Build history of the part. All positions in model axes, mm. A direction names the side the tool comes from. Give positions to 0.01 mm unless a question says otherwise; leave off trailing zeros. Write each loop counter-clockwise with the first axis right and the second up, starting at its lowest first coordinate (ties: lowest second). Pieces come first, ordered by that corner, then holes. Notation, with made-up numbers: (-13.75, 73) -> (28.25, 73) arc R16 cw to (28.25, 85) -> close; hole circle Ø1 at (-30, 49). An arc over 180 degrees is marked (long way). Put each result on its own line as item: value. Start each with the question number.
Item 1: Two-plate mould, pull along Y, no slides. Class faces 1 (the flat face through (-25, 19.05, 3)), 2 (the flat face through (-25, 76.2, 3)), 3 (the flat face through (-30.162, 13, 3)), 4 (the flat face through (-50.8, 38, 3)): pulls with the +Y half, pulls with the -Y half, needs draft (parallel to the pull), parting line crosses it, or undercut.
Item 2: Slice it at B-B, the plane x = -22.5. List the corners of the cut face in (y, z).
Item 3: Tool access for faces 5 (the flat face through (-26, 38, 0)), 6 (the flat face through (-30.162, 63, 3)): list every direction of +Z, -Z, +X, -X, +Y, -Y with a clear straight run to the whole face (end or side of a thin tool).
Item 4: Slice it at C-C, the plane z = 3. List the corners of the cut face in (x, y), plus the area to 3 significant figures.
Item 5: Slice it at A-A, the plane y = 13.5. List the corners of the cut face in (x, z).
Item 6: Drill centre lines: line 1 along Y through (x, z) = (-23.5, 5.5); line 2 along X through (y, z) = (57.5, 1.25). Where is each one in solid material? Low to high.
Item 7: Flat gauge pin, fed straight in: pin 1 Ø1.9 at (x, z) = (-26, 3) entering from -Y. Where does the tip first touch, or does it go through?
```python
from build123d import *

# Parameters (mm, degrees)
SKETCH1_W           = 76.2
SKETCH1_H           = 50.8
BOSS_EXTRUDE1_DEPTH = 6.35
SKETCH2_W           = 9.525
SKETCH2_H           = 12.7
CUT_EXTRUDE1_DEPTH  = 92.800885072


with BuildPart() as part:
    # Sketch1 → Boss-Extrude1 (new body)
    with BuildSketch(Plane(origin=(0, 0, 0), x_dir=(0, 1, 0), z_dir=(0, 0, 1))):
        with Locations((38.1, 25.4)):
            Rectangle(SKETCH1_W, SKETCH1_H)
    extrude(amount=BOSS_EXTRUDE1_DEPTH)

    # Sketch2 → Cut-Extrude1 (cut, through all)
    with BuildSketch(Plane.XY.offset(6.35)):
        with Locations((-25.4, 12.7)):
            Rectangle(SKETCH2_W, SKETCH2_H)
        with Locations((-25.4, 63.5)):
            Rectangle(SKETCH2_W, SKETCH2_H)
    extrude(amount=-CUT_EXTRUDE1_DEPTH, mode=Mode.SUBTRACT)


solid = part.part
```
Values follow:
1. face 1: undercut
1. face 2: pulls with the +Y half
1. face 3: undercut
1. face 4: needs draft
2. outline: (0, 0) -> (6.35, 0) -> (6.35, 6.35) -> (0, 6.35) -> close; (19.05, 0) -> (57.15, 0) -> (57.15, 6.35) -> (19.05, 6.35) -> close; (69.85, 0) -> (76.2, 0) -> (76.2, 6.35) -> (69.85, 6.35) -> close
3. face 5: -Z, +X, -X, +Y, -Y
3. face 6: +Z, -Z
4. outline: (-50.8, 0) -> (0, 0) -> (0, 76.2) -> (-50.8, 76.2) -> close; hole (-30.16, 6.35) -> (-20.64, 6.35) -> (-20.64, 19.05) -> (-30.16, 19.05) -> close; hole (-30.16, 57.15) -> (-20.64, 57.15) -> (-20.64, 69.85) -> (-30.16, 69.85) -> close
4. area: 3,630 mm2
5. outline: (-50.8, 0) -> (-30.16, 0) -> (-30.16, 6.35) -> (-50.8, 6.35) -> close; (-20.64, 0) -> (0, 0) -> (0, 6.35) -> (-20.64, 6.35) -> close
6. line 1: 0 to 6.35, 19.05 to 57.15, 69.85 to 76.2
6. line 2: -50.8 to -30.16, -20.64 to 0
7. pin 1: y = 0
